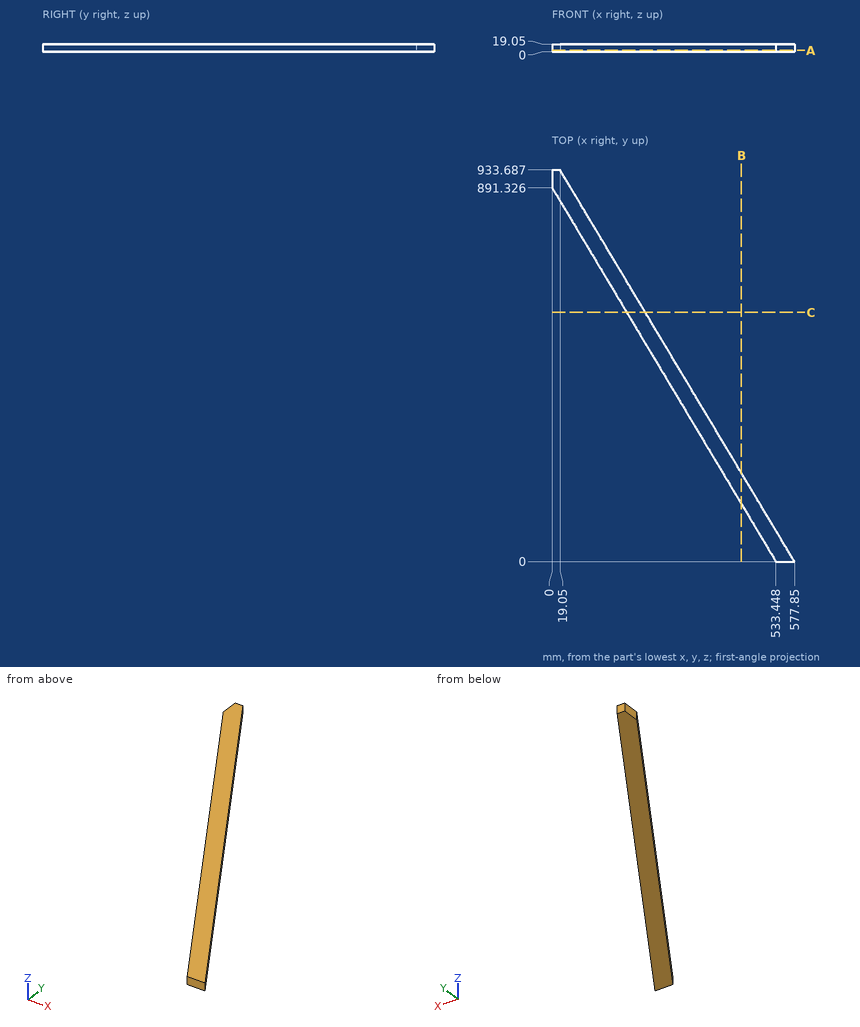
Geometry check sheet. Reference: drawing and pictorial views, mm from the part's lowest x, y, z. Round coordinates to 2 decimals unless told otherwise and drop trailing zeros. Loops run counter-clockwise (first coordinate to the right, second up) from the corner with the lowest first, then second, coordinate; pieces in that order, holes last. Notation, with made-up numbers: (-5.5, 47) -> (44.5, 47) arc R23 cw to (44.5, 63) -> close; hole circle Ø5 at (-5, 85). An arc over 180 degrees is marked (long way). Answer as a JSON object with one key per item and string values. Group by question number.
Item 1: Thickness scan on line 1 along X through (y, z) = (785, 3) (1 decimal); line 2 along Y through (x, z) = (119, 17); line 3 along Y through (x, z) = (449.5, 7.5) (1 decimal). Record the ranges inside material, lowest first.
Item 2: Cross-section at B-B, the plane x = 451. Record the cut outline in (y, z).
Item 3: Cross-section at A-A, the plane z = 4. Record the cut outline in (x, y).
Item 4: Cross-section at C-C, the plane y = 594.5. Record the cut outline in (x, z).
Item 5: Depth check by flat-ended pin: pin 1 Ø5 at (y, z) = (102.5, 9) entering from +X; pin 2 Ø2 at (x, z) = (98, 13.5) entering from +Y; pin 3 Ø2 at (x, z) = (205, 15.5) entering from +Y. Enter the tip coordinate at first touch or a pass-through.
Determined:
{
 "1": {"line 1": "x = 63.6 to 108", "line 2": "y = 692.49 to 766.68", "line 3": "y = 140.3 to 214.5"},
 "2": {"outline": "(137.76, 0) -> (211.95, 0) -> (211.95, 19.05) -> (137.76, 19.05) -> close"},
 "3": {"outline": "(0, 891.33) -> (533.45, 0) -> (577.85, 0) -> (19.05, 933.69) -> (0, 933.69) -> close"},
 "4": {"outline": "(177.65, 0) -> (222.05, 0) -> (222.05, 19.05) -> (177.65, 19.05) -> close"},
 "5": {"pin 1": "stops at x = 518", "pin 2": "stops at y = 803.44", "pin 3": "stops at y = 624.66"}
}
